Source: CAD feature listing. Evaluate the final solid. Frame: model axes, mm. A direction names the side the tool comes from. Coordinates: 2 decimals unless noted, no trailing zeros. Write each loop counter-clockwise with the first axis right and the second up, starting at its lowest first coordinate (ties: lowest second). Pieces come first, ordered by that corner, then holes. Notation, with made-up numbers: (-23, 45) - (18, 45) arc R13 ccw to (18, 68) - close; hole circle Ø1 at (79, 85.5). An arc over 180 degrees is marked (long way). One line per item, written item: value.
from build123d import *

# Parameters (mm, degrees)
F0_R     = 200
F1_DEPTH = 2
F2_R     = 75
F3_DEPTH = 150


with BuildPart() as f1:
    # F0 (on Top) → F1 (new body)
    with BuildSketch(Plane.XY):
        Circle(F0_R)
    extrude(amount=F1_DEPTH)

    # F2 (on face) → F3 (join)
    with BuildSketch(Plane.XY.offset(2)):
        Circle(F2_R)
    extrude(amount=F3_DEPTH)

    # F4: F1 across face


with BuildPart() as f1_1:
    add(f1.part)
    add(f1.part.mirror(Plane(origin=(0, 0, 0), x_dir=(1, 0, 0), z_dir=(0, 0, -1))))


solid = f1_1.part
1) Section query D-D on y = -175.5. Output: boundary loops of the cut face in (x, z).
Values found:
outline: (-95.92, -2) - (95.92, -2) - (95.92, 2) - (-95.92, 2) - close
2) Section query A-A on y = 0. Output: boundary loops of the cut face in (x, z), then the cut area to 3 significant figures.
Values found:
outline: (-200, -2) - (-75, -2) - (-75, -152) - (75, -152) - (75, -2) - (200, -2) - (200, 2) - (75, 2) - (75, 152) - (-75, 152) - (-75, 2) - (-200, 2) - close
area: 46,600 mm2
3) Material intervals for line 1 (Z direction, x = 129.5, y = 110); line 2 (Y direction, x = 3, z = 18); line 3 (X direction, y = -62, z = 116), sorted ascending.
Values found:
line 1: -2 to 2
line 2: -74.94 to 74.94
line 3: -42.2 to 42.2
4) Reachability of faces 1 (the flat face through (-1, 1, 152)), 2 (the cylindrical face through (-9.764, 74.362, -75.95)), 3 (the flat face through (-3, -86, 2)) from +Z, -Z, +X, -X, +Y, -Y: full face, straight path, thin tool, end or side. Return the list, or none.
Values found:
face 1: +Z, +X, -X, +Y, -Y
face 2: -Z
face 3: +Z
5) Contact query for flat-ended pins moving along their axis: P1, Ø6, axis at x = 127.5, y = -107, coming from the -Z side; P2, Ø1, axis at x = 60.5, y = -108.5, coming from the +Z side. Output: stop coordinate, or through.
Values found:
P1: z = -2
P2: z = 2
6) Section query C-C on z = -119.5. Output: boundary loops of the cut face in (x, y).
Values found:
outline: circle Ø150 at (0, 0)
